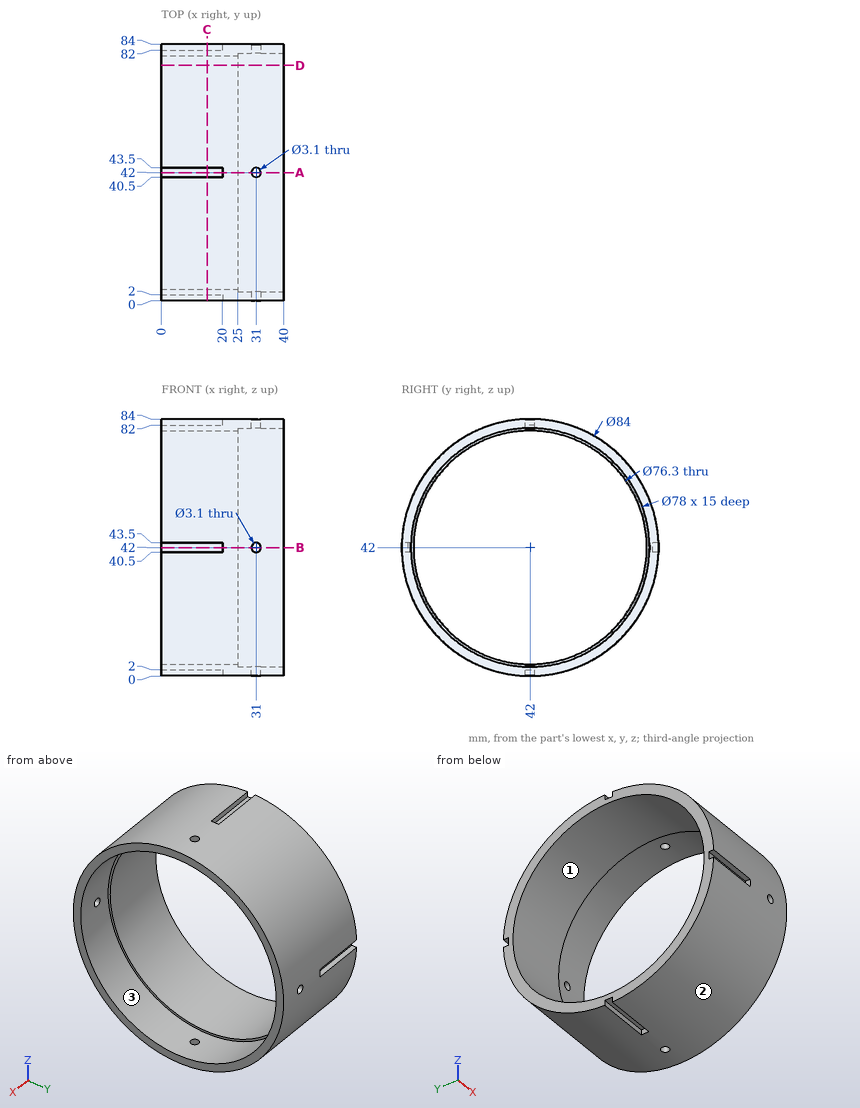
The drawing under review shows one solid part. Ordinate dimensions are in mm from its lowest x, y, z. Give positions to 0.01 mm unless a question says otherwise; leave off trailing zeros. Order: outer loops, then holes, each group sorted by start corner. A loop starts at its lowest first (then second) coordinate and runs counter-clockwise, first axis right, second up. Notation, with made-up numbers: M 26.25,64.5 L 80.25,64.5 A11 ccw 80.25,78.5 Z; hole C 82.5,-8.5 d8. An arc over 180 degrees is marked long. One line per question, with ' | ' between items. Start each with the question number.
Q1. We need section C-C (x = 15). Write out the cut boundary in (y, z).
Q2. We need section D-D (y = 77). Write out the cut boundary in (x, z), plus the area to 3 significant figures.
Q3. For pin 1 Ø1.6 at (y, z) = (42.5, 82.5) entering from -X; pin 2 Ø10 at (x, y) = (29, 31) entering from -Z; pin 3 Ø5 at (x, y) = (20, 27.5) entering from -Z; pin 4 Ø5 at (x, z) = (27, 47) entering from -Y, all flat-tipped, find the tip position at first contact; note any pin that passes through.
Q4. We need section A-A (y = 42). Write out the cut boundary in (x, z), plus the area to 3 significant figures.
Q5. The part is to be moulded in two halves that separate along Z. For the marked faces 1, 2 and 3, say which applies: +Z half, -Z half, draft (parallel to the pull), parting line (faces both ways), or undercut.
Q6. For L1, parallel to Y at x = 19, z = 41; L2, parallel to X at y = 42, z = 83.1; L3, parallel to Z at x = 22, y = 13, list the stretches that pass through material, from the lowest coordinate up. Write a range as [from, to].
Returned:
1) outline: M 0.03,40.5 A42 ccw 40.5,0.03 L 40.5,2 L 43.5,2 L 43.5,0.03 A42 ccw 83.97,40.5 L 82,40.5 L 82,43.5 L 83.97,43.5 A42 ccw 43.5,83.97 L 43.5,82 L 40.5,82 L 40.5,83.97 A42 ccw 0.03,43.5 L 2,43.5 L 2,40.5 Z; hole C 42,42 d76.3
2) outline: M 0,18.78 L 40,18.78 L 40,24.8 L 25,24.8 L 25,26.82 L 0,26.82 Z; M 0,57.18 L 25,57.18 L 25,59.2 L 40,59.2 L 40,65.22 L 0,65.22 Z | area: 582 mm2
3) pin 1: x = 0 | pin 2: z = 0.43 | pin 3: z = 1.75 | pin 4: y = 0.07
4) outline: M 0,2 L 20,2 L 20,0 L 29.45,0 L 29.45,3 L 25,3 L 25,3.85 L 0,3.85 Z; M 0,80.15 L 25,80.15 L 25,81 L 29.45,81 L 29.45,84 L 20,84 L 20,82 L 0,82 Z; M 32.55,0 L 40,0 L 40,3 L 32.55,3 Z; M 32.55,81 L 40,81 L 40,84 L 32.55,84 Z | area: 184 mm2
5) face 1: undercut | face 2: parting line | face 3: undercut
6) L1: [2, 3.86], [80.14, 82] | L2: [20, 29.45], [32.55, 40] | L3: [11.62, 17.21], [66.79, 72.38]
